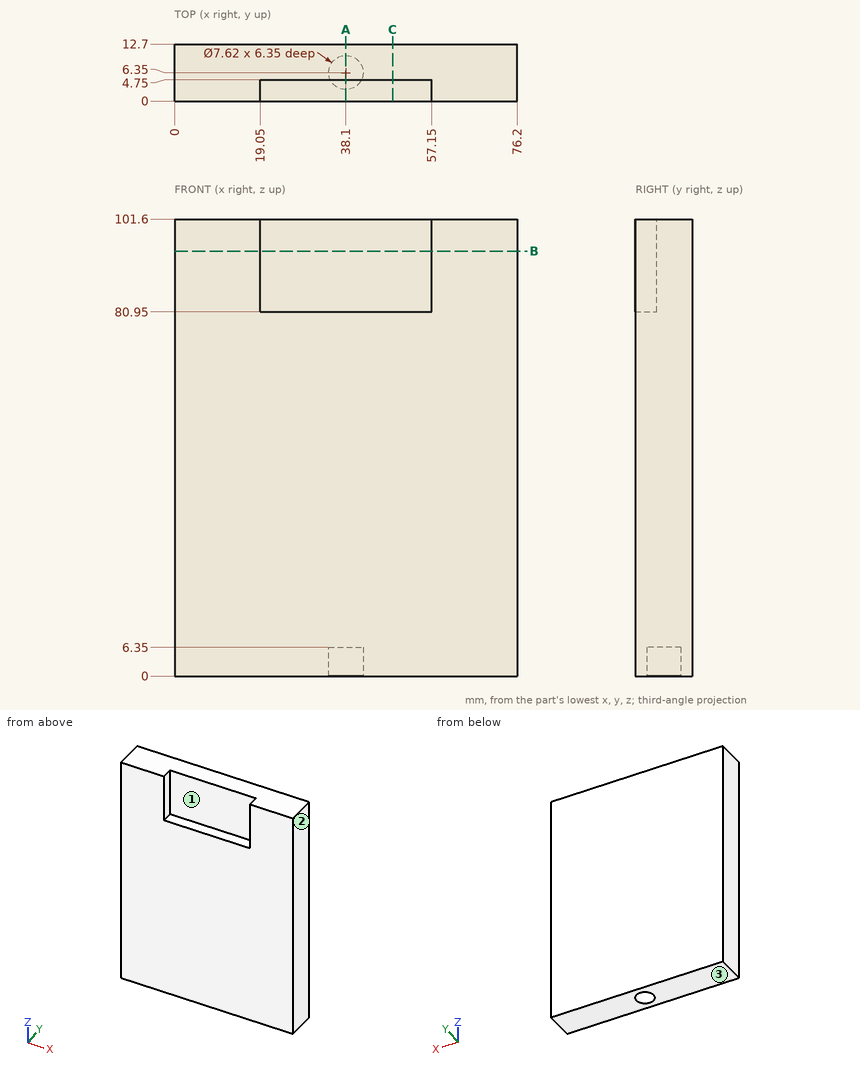
For this review, use the dimensioned drawing (mm, ordinates from the lowest corner) and the shaded views. Round coordinates to 2 decimals unless told otherwise and drop trailing zeros. Order: outer loops, then holes, each group sorted by start corner. A loop starts at its lowest first (then second) coordinate and runs counter-clockwise, first axis right, second up. Notation, with made-up numbers: M 43,42.5 L 92,42.5 A13 cw 92,51.5 Z; hole C 66,65.25 d3. An arc over 180 degrees is marked long. Write each question's results on one line, items separated by ' | '. Start each with the question number.
1. Clearance check with flat-ended pins moving along their axes: pin 1 Ø6 at (x, y) = (37.5, 8) entering from -Z; pin 2 Ø1.4 at (x, y) = (38, 2.5) entering from +Z. State where each tip first meets the part, or that it passes through.
2. Add section B-B (z = 94.5). State the section outline as (x, y) points.
3. Add section C-C (x = 48.5). State the section outline as (y, z) points, then the cut area to 3 significant figures.
4. To check wall thickness, follow L1, parallel to Y at x = 38.1, z = 4.5; L2, parallel to X at y = 2, z = 93; L3, parallel to Z at x = 32, y = 4. State the ranges of each line that lie inside material, in increasing order. Write a range as [from, to].
5. Draft analysis for pull direction X (two halves, no side actions). For the marked faces 1, 2 and 3, state which applies: pulls with the +X half, pulls with the -X half, needs draft (parallel to the pull), parting line crosses it, or undercut.
6. Add section A-A (x = 38.1). State the section outline as (y, z) points, then the cut area to 3 significant figures.
Output values:
1) pin 1: z = 0 | pin 2: z = 80.95
2) outline: M 0,0 L 19.05,0 L 19.05,4.75 L 57.15,4.75 L 57.15,0 L 76.2,0 L 76.2,12.7 L 0,12.7 Z
3) outline: M 0,0 L 12.7,0 L 12.7,101.6 L 4.75,101.6 L 4.75,80.95 L 0,80.95 Z | area: 1,190 mm^2
4) L1: [0, 2.54], [10.16, 12.7] | L2: [0, 19.05], [57.15, 76.2] | L3: [0, 80.95]
5) face 1: undercut | face 2: pulls with the +X half | face 3: needs draft
6) outline: M 0,0 L 2.54,0 L 2.54,6.35 L 10.16,6.35 L 10.16,0 L 12.7,0 L 12.7,101.6 L 4.75,101.6 L 4.75,80.95 L 0,80.95 Z | area: 1,140 mm^2
